Read the model definition and answer for the solid it produces. Units are mm, in the model's axes. Face numbers are marked on the shaded views. A direction names the side the tool comes from. Round coordinates to 2 decimals unless told otherwise and drop trailing zeros. Loops run counter-clockwise (first coordinate to the right, second up) from the corner with the lowest first, then second, coordinate; pieces in that order, holes last. Notation, with made-up numbers: (-7, 25.5) - (11, 25.5) arc R15 ccw to (11, 30.5) - close; hole circle Ø10 at (13, 58.5). An arc over 180 degrees is marked (long way). Answer as CSV lines item,"result".
```python
from build123d import *

# Parameters (mm, degrees)
EXTRUDE_1_DEPTH = 1.2
MM_1_D          = 2.5
SKETCH_4_W      = 6.6
SKETCH_4_H      = 23.6
SKETCH_4_W_2    = 4.5
SKETCH_4_H_2    = 9
SKETCH_4_W_3    = 5.3
SKETCH_4_H_3    = 7.5
EXTRUDE_2_DEPTH = 2
SKETCH_5_W      = 11
SKETCH_5_H      = 15
EXTRUDE_3_DEPTH = 6.3


with BuildPart() as part:
    # 草图1 → 凸台-拉伸1 (new body)
    with BuildSketch(Plane(origin=(0, 0, 0), x_dir=(1, 0, 0), z_dir=(0, 1, 0))):
        with BuildLine():
            Line((-26.32, -32.825), (26.32, -32.825))
            ThreePointArc((26.32, -32.825), (27.734213562, -32.239213562), (28.32, -30.825))
            Line((28.32, -30.825), (28.32, 30.825))
            ThreePointArc((28.32, 30.825), (27.734213562, 32.239213562), (26.32, 32.825))
            Line((26.32, 32.825), (-26.32, 32.825))
            ThreePointArc((-26.32, 32.825), (-27.734213562, 32.239213562), (-28.32, 30.825))
            Line((-28.32, 30.825), (-28.32, -30.825))
            ThreePointArc((-28.32, -30.825), (-27.734213562, -32.239213562), (-26.32, -32.825))
        make_face()
    extrude(amount=EXTRUDE_1_DEPTH)

    # 大小mm 暗销孔1 (through all)
    with Locations(Plane(origin=(0, 1.2, 0), x_dir=(1, 0, 0), z_dir=(0, 1, 0))):
        with Locations((-25.82, 30.325), (-25.82, -30.325), (25.82, -30.325), (25.82, 30.325)):
            Hole(MM_1_D / 2)

    # 草图4 → 凸台-拉伸2 (add)
    with BuildSketch(Plane(origin=(0, 1.2, 0), x_dir=(1, 0, 0), z_dir=(0, 1, 0))):
        with Locations((-18.52, -5.675)):
            Rectangle(SKETCH_4_W, SKETCH_4_H)
        with Locations((-19.57, 22.625)):
            Rectangle(SKETCH_4_W_2, SKETCH_4_H_2)
        with Locations((27.43, 5.075)):
            Rectangle(SKETCH_4_W_3, SKETCH_4_H_3)
    extrude(amount=EXTRUDE_2_DEPTH)

    # 草图5 → 凸台-拉伸3 (add)
    with BuildSketch(Plane(origin=(0, 1.2, 0), x_dir=(1, 0, 0), z_dir=(0, 1, 0))):
        with Locations((24.32, -14.325)):
            Rectangle(SKETCH_5_W, SKETCH_5_H)
    extrude(amount=EXTRUDE_3_DEPTH)


solid = part.part
```
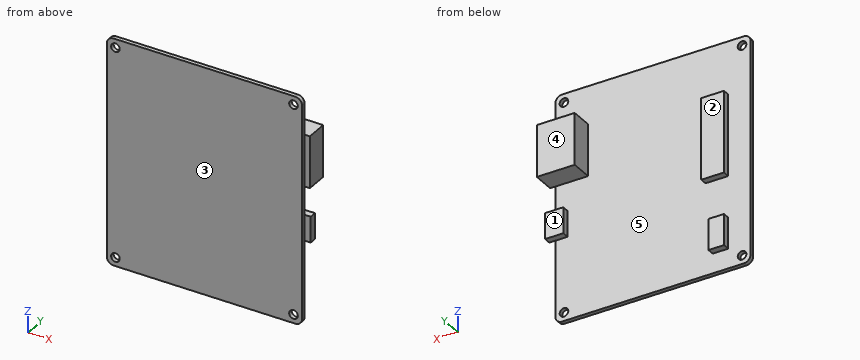
1) A tool of negligible diameter and unlimited length cuts with its end or side. For the marked faces 1, 2 and 3, from which of +Z, -Z, +X, -X, +Y, -Y can it reach the whole face along a straight path? Write none if from no direction.
Entries:
face 1,"-Z, +X, -X, +Y"
face 2,"+Z, -Z, -X, +Y"
face 3,"+Z, -Z, +X, -X, -Y"
2) Find the intervals of material crossed by line 1 (Z direction, x = -25.82, y = 0.35) (3 decimals); line 2 (Z direction, x = 26, y = 1.5) (3 decimals); line 3 (Y direction, x = -4, z = 10), in increasing order.
Entries:
line 1,"z = -32.825 to -31.575, -29.075 to 29.075, 31.575 to 32.825"
line 2,"z = -8.825 to -1.325, 6.825 to 21.825"
line 3,"y = 0 to 1.2"
3) A cutting plane is placed at B-B, the plane y = 6.5. Determine the outline of the cut face in (x, z) (3 decimals).
Entries:
outline,"(18.82, 6.825) - (29.82, 6.825) - (29.82, 21.825) - (18.82, 21.825) - close"
4) The mould has two halves that part along X. Classify the marked faces 4 and 5: pulls with the +X half, pulls with the -X half, needs draft (parallel to the pull), parting line crosses it, or undercut.
Entries:
face 4,"needs draft"
face 5,"undercut"
5) A cutting plane is placed at C-C, the plane z = -28. Determine the outline of the cut face in (x, y).
Entries:
outline,"(-28.32, 0) - (28.32, 0) - (28.32, 1.2) - (-28.32, 1.2) - close"
6) Each of these flat-tipped pins is pushed along its axis until it touches: P1, Ø2, axis at y = 2, z = -21.5, coming from the -X side; P2, Ø0.6, axis at y = 0.5, z = -12, coming from the +X side; P3, Ø1, axis at x = -19, y = 2, coming from the +Z side (3 decimals); P4, Ø7.5, axis at x = -17, z = 11, coming from the +Y side. Where does it stop, or does it pass through?
Entries:
P1,"stops at x = -28.32"
P2,"stops at x = 28.32"
P3,"stops at z = 17.475"
P4,"stops at y = 3.2"
7) A cutting plane is placed at A-A, the plane x = 23. Determine the outline of the cut face in (y, z) (3 decimals).
Entries:
outline,"(0, -32.825) - (1.2, -32.825) - (1.2, 6.825) - (7.5, 6.825) - (7.5, 21.825) - (1.2, 21.825) - (1.2, 32.825) - (0, 32.825) - close"
